The listing builds one solid part. Answer for the finished solid, in the listing's coordinates (mm). Round coordinates to 2 decimals unless told otherwise and drop trailing zeros. Loops run counter-clockwise (first coordinate to the right, second up) from the corner with the lowest first, then second, coordinate; pieces in that order, holes last. Notation, with made-up numbers: (37, 76.5) - (58, 76.5) arc R24 cw to (58, 89.5) - close; hole circle Ø6 at (-11.5, 14). An arc over 180 degrees is marked (long way). Write item = value, one per line. Start each with the question number.
1) Given pin 1 Ø6.5 at (x, z) = (-47.4, -12.52) entering from +Y; pin 2 Ø4 at (x, z) = (25.4, 0) entering from -Y; pin 3 Ø3 at (y, z) = (5, -81.5) entering from +X; pin 4 Ø1 at (x, y) = (13, 1.5) entering from +Z, each flat-ended and moving along its own axis, determine where each tip first touches the part or whether it passes through.
2) For a pull along Z with two mould halves and no side action, classify faces 1 (the cylindrical face through (-53.247, 3.131, -78.85)), 2 (the cylindrical face through (0.32, 3.13, 29.97)), 3 (the cylindrical face through (-20.335, 3.131, 17.213)) as released by +Z, released by -Z, zero draft, split by the parting line, or undercut.
3) Section D-D, the plane x = 0 is taken. Determine the outline of the cut face in (y, z) (3 decimals), and give its area (3 significant figures).
4) Section B-B, the plane x = -18 is taken. Determine the outline of the cut face in (y, z) (3 decimals).
5) Section A-A, the plane z = -94 is taken. Determine the outline of the cut face in (x, y), and give its area (3 significant figures).
6) Straight lines are drawn through the part: line 1 along X through (y, z) = (5, -18); line 2 along Z through (x, y) = (0, 2.75) (3 decimals); line 3 along Z through (x, y) = (26, 1). For each, find the intervals that lie inside material, in ascending order.
7) Section C-C, the plane z = 0 is taken. Determine the outline of the cut face in (x, y) (3 decimals), and give its area (3 significant figures).
Autodesk Inventor part; units mm, degrees
ref_plane "YZ Plane" through (0, 0, 0) normal (1, 0, 0) x (0, 1, 0)
ref_plane "XZ Plane" through (0, 0, 0) normal (0, 1, 0) x (-1, 0, 0)
ref_plane "XY Plane" through (0, 0, 0) normal (0, 0, 1) x (1, 0, 0)
sketch "Sketch1" plane through (0, 0, 0) normal (0, 1, 0) x (-1, 0, 0)
  point P0 (0, 0)
sketch "Sketch2" plane through (0, 0, 0) normal (0, 1, 0) x (-1, 0, 0)
  circle A0 centre (0, 0) radius 6.35 construction
  circle A1 centre (0, -44.45) radius 38.1 construction
  circle A2 centre (0, 0) radius 25.4 construction
  circle A3 centre (17.9605, -17.9605) radius 2.4892
  circle A4 centre (25.4, 0) radius 2.4892
  circle A5 centre (17.9605, 17.9605) radius 2.4892
  circle A6 centre (0, 25.4) radius 2.4892
  circle A7 centre (-17.9605, 17.9605) radius 2.4892
  circle A8 centre (-25.4, 0) radius 2.4892
  circle A9 centre (-17.9605, -17.9605) radius 2.4892
  circle A10 centre (0, -25.4) radius 2.4892 construction
  circle A11 centre (0, -88.9) radius 25.4 construction
  circle A12 centre (0, -88.9) radius 6.35 construction
  circle A13 centre (-17.9605, -70.9395) radius 2.4892
  circle A14 centre (-25.4, -88.9) radius 2.4892
  circle A15 centre (-17.9605, -106.8605) radius 2.4892
  circle A16 centre (0, -114.3) radius 2.4892
  circle A17 centre (17.9605, -106.8605) radius 2.4892
  circle A18 centre (25.4, -88.9) radius 2.4892
  circle A19 centre (17.9605, -70.9395) radius 2.4892
  circle A20 centre (0, -63.5) radius 2.4892 construction
  circle A21 centre (0, 0) radius 9.525
  circle A22 centre (0, -88.9) radius 9.525
  circle A23 centre (47.3968, -12.5178) radius 6.35 construction
  circle A24 centre (47.3968, -76.3822) radius 6.35 construction
  circle A25 centre (-47.3968, -76.3822) radius 6.35 construction
  circle A26 centre (0, 0) radius 29.972 construction
  circle A27 centre (0, -88.9) radius 29.972 construction
  circle A28 centre (-47.3968, -12.5178) radius 6.35 construction
  circle A29 centre (47.3968, -12.5178) radius 2.0193
  circle A30 centre (47.3968, -76.3822) radius 2.0193
  circle A31 centre (-47.3968, -12.5178) radius 2.0193
  circle A32 centre (-47.3968, -76.3822) radius 2.0193
  line L0 (42.1305, -72.8341) -> (31.5979, -65.7381) construction
  line L1 (41.2573, -78.0036) -> (28.9784, -81.2466) construction
  line L2 (-41.2573, -78.0036) -> (-28.9784, -81.2466) construction
  line L3 (-42.1305, -72.8341) -> (-31.5979, -65.7381) construction
  line L4 (-41.2573, -10.8964) -> (-28.9784, -7.6534) construction
  line L5 (-42.1305, -16.0659) -> (-31.5979, -23.1619) construction
  line L6 (41.2573, -10.8964) -> (28.9784, -7.6534) construction
  line L7 (42.1305, -16.0659) -> (31.5979, -23.1619) construction
  line L8 (-20.6699, 21.7043) -> (-51.7761, -7.9195)
  line L9 (-53.7468, -12.5178) -> (-53.7468, -76.3822)
  line L10 (-51.7761, -80.9805) -> (-20.6699, -110.6043)
  line L11 (20.6699, -110.6043) -> (51.7761, -80.9805)
  line L12 (53.7468, -76.3822) -> (53.7468, -12.5178)
  line L13 (51.7761, -7.9195) -> (20.6699, 21.7043)
  arc A33 (20.6699, 21.7043) -> (-20.6699, 21.7043) centre (0, 0) ccw
  arc A34 (-51.7761, -7.9195) -> (-53.7468, -12.5178) centre (-47.3968, -12.5178) ccw
  arc A35 (-53.7468, -76.3822) -> (-51.7761, -80.9805) centre (-47.3968, -76.3822) ccw
  arc A36 (-20.6699, -110.6043) -> (20.6699, -110.6043) centre (0, -88.9) ccw
  arc A37 (51.7761, -80.9805) -> (53.7468, -76.3822) centre (47.3968, -76.3822) ccw
  arc A38 (53.7468, -12.5178) -> (51.7761, -7.9195) centre (47.3968, -12.5178) ccw
  circle A39 centre (0, -44.45) radius 14.351
  dimension "d2" = 50.8
  dimension "d0" = 12.7
  dimension "d1" = 76.2
  dimension "d3" = 4.9784
  dimension "d6" = 360
  dimension "d8" = 4.9784
  dimension "d11" = 360
  dimension "d13" = 19.05
  dimension "d14" = 19.05
  dimension "d15" = 59.944
  dimension "d16" = 59.944
  dimension "d17" = 12.7
  dimension "d18" = 4.0386
  dimension "d24" = 12.7
  dimension "d25" = 28.702
extrude "Extrusion1" add sketch "Sketch2" along normal blind 6.35
properties part number "Bottom Plate"
Geometry check:
q1.pin_1 = 6.35
q1.pin_2 = through
q1.pin_3 = 52.62
q1.pin_4 = 27.24
q2.face_1 = released by -Z
q2.face_2 = released by +Z
q2.face_3 = undercut
q3.outline = (0, -118.872) - (6.35, -118.872) - (6.35, -116.789) - (0, -116.789) - close; (0, -111.811) - (6.35, -111.811) - (6.35, -98.425) - (0, -98.425) - close; (0, -79.375) - (6.35, -79.375) - (6.35, -58.801) - (0, -58.801) - close; (0, -30.099) - (6.35, -30.099) - (6.35, -9.525) - (0, -9.525) - close; (0, 9.525) - (6.35, 9.525) - (6.35, 22.911) - (0, 22.911) - close; (0, 27.889) - (6.35, 27.889) - (6.35, 29.972) - (0, 29.972) - close
q3.area = 458 mm2
q4.outline = (0, -112.865) - (6.35, -112.865) - (6.35, -109.349) - (0, -109.349) - close; (0, -104.372) - (6.35, -104.372) - (6.35, -73.428) - (0, -73.428) - close; (0, -68.451) - (6.35, -68.451) - (6.35, -20.449) - (0, -20.449) - close; (0, -15.472) - (6.35, -15.472) - (6.35, 15.472) - (0, 15.472) - close; (0, 20.449) - (6.35, 20.449) - (6.35, 23.965) - (0, 23.965) - close
q5.outline = (-38.11, 0) - (-8.04, 0) - (-8.04, 6.35) - (-38.11, 6.35) - close; (8.04, 0) - (38.11, 0) - (38.11, 6.35) - (8.04, 6.35) - close
q5.area = 382 mm2
q6.line_1 = -53.75 to -20.45, -15.47 to 15.47, 20.45 to 53.75
q6.line_2 = -118.872 to -116.789, -111.811 to -98.425, -79.375 to -58.801, -30.099 to -9.525, 9.525 to 22.911, 27.889 to 29.972
q6.line_3 = -105.53 to -91.32, -86.48 to -2.42, 2.42 to 16.63
q7.outline = (-43.46, 0) - (-27.889, 0) - (-27.889, 6.35) - (-43.46, 6.35) - close; (-22.911, 0) - (-9.525, 0) - (-9.525, 6.35) - (-22.911, 6.35) - close; (9.525, 0) - (22.911, 0) - (22.911, 6.35) - (9.525, 6.35) - close; (27.889, 0) - (43.46, 0) - (43.46, 6.35) - (27.889, 6.35) - close
q7.area = 368 mm2
